The model under review builds one solid part; all positions refer to its coordinate system, in mm. A direction names the side the tool comes from. Round coordinates to 2 decimals unless told otherwise and drop trailing zeros. Order: outer loops, then holes, each group sorted by start corner. A loop starts at its lowest first (then second) coordinate and runs counter-clockwise, first axis right, second up.
```python
from build123d import *

# Parameters (mm, degrees)
SKETCH1_W           = 50
SKETCH1_H           = 77.4
SKETCH1_R           = 2
BOSS_EXTRUDE1_DEPTH = 4
SKETCH2_W           = 50
SKETCH2_H           = 7.168288369
BOSS_EXTRUDE2_DEPTH = 60
SKETCH6_W           = 20
SKETCH6_H           = 26
CUT_EXTRUDE1_DEPTH  = 124.730240351
RIB1_REACH          = 97.821
SKETCH7_WALL_W      = 250.948466038
SKETCH7_WALL_H      = 14
FILLET2_R           = 2
FILLET3_R           = 12
SKETCH8_W           = 13
SKETCH8_H           = 7.168288369
BOSS_EXTRUDE3_DEPTH = 20
FILLET4_R           = 4
BOSS_EXTRUDE4_DEPTH = 6
FILLET5_R           = 2


with BuildPart() as part:
    # Sketch1 → Boss-Extrude1 (new body)
    with BuildSketch(Plane.ZY.offset(8)):
        with Locations((55.110705908, 0)):
            Rectangle(SKETCH1_W, SKETCH1_H)
        with Locations((34.110705908, 33.7)):
            Circle(SKETCH1_R, mode=Mode.SUBTRACT)
        with Locations((41.110705908, 33.7)):
            Circle(SKETCH1_R, mode=Mode.SUBTRACT)
        with Locations((69.110705908, 33.7)):
            Circle(SKETCH1_R, mode=Mode.SUBTRACT)
        with Locations((76.110705908, 33.7)):
            Circle(SKETCH1_R, mode=Mode.SUBTRACT)
        with Locations(Location((34.110705908, -33.7, 0), (0, 0, 180))):
            Circle(SKETCH1_R, mode=Mode.SUBTRACT)
        with Locations(Location((41.110705908, -33.7, 0), (0, 0, 180))):
            Circle(SKETCH1_R, mode=Mode.SUBTRACT)
        with Locations(Location((69.110705908, -33.7, 0), (0, 0, 180))):
            Circle(SKETCH1_R, mode=Mode.SUBTRACT)
        with Locations(Location((76.110705908, -33.7, 0), (0, 0, 180))):
            Circle(SKETCH1_R, mode=Mode.SUBTRACT)
    extrude(amount=BOSS_EXTRUDE1_DEPTH)

    # Sketch2 → Boss-Extrude2 (add)
    with BuildSketch(Plane.ZY.offset(12)):
        with Locations((55.110705908, -25.772954127)):
            Rectangle(SKETCH2_W, SKETCH2_H)
    extrude(amount=BOSS_EXTRUDE2_DEPTH)

    # Sketch6 → Cut-Extrude1 (cut, through all)
    with BuildSketch(Plane(origin=(0, -22.188809942, 0), x_dir=(1, 0, 0), z_dir=(0, 1, 0))):
        with Locations((-22, -43.110705908)):
            Rectangle(SKETCH6_W, SKETCH6_H)
    extrude(amount=-CUT_EXTRUDE1_DEPTH, mode=Mode.SUBTRACT)

    # Sketch7 wall → Rib1 (add, up to next)
    with BuildSketch(Plane(origin=(-26, 2.811190058, 80.110705908), x_dir=(0.488603368932, 0.87250601595, 0), z_dir=(-0.87250601595, 0.488603368932, 0)), mode=Mode.PRIVATE) as rib1_sk1:
        with Locations((0, 7)):
            Rectangle(SKETCH7_WALL_W, SKETCH7_WALL_H)
    rib1_tool1 = extrude(rib1_sk1.sketch, amount=-RIB1_REACH, mode=Mode.PRIVATE) - part.part
    add(rib1_tool1.solids().sort_by_distance((-26, 2.811190058, 80.110705908))[0])

    # Fillet2
    fillet2_edges = [part.edges().sort_by_distance(p)[0] for p in [
        (-12, -29.357098311, 68.110705908),
    ]]
    fillet(fillet2_edges, radius=FILLET2_R)

    # Fillet3
    fillet3_edges = [part.edges().sort_by_distance(p)[0] for p in [
        (-32, -25.772954126, 56.110705908),
    ]]
    fillet(fillet3_edges, radius=FILLET3_R)

    # Sketch8 → Boss-Extrude3 (add)
    with BuildSketch(Plane(origin=(-32, 0, 0), x_dir=(0, 0, -1), z_dir=(1, 0, 0))):
        with Locations((-36.610705908, -25.772954127)):
            Rectangle(SKETCH8_W, SKETCH8_H)
    extrude(amount=BOSS_EXTRUDE3_DEPTH)

    # Fillet4
    fillet4_edges = [part.edges().sort_by_distance(p)[0] for p in [
        (-32, -25.772954126, 43.110705908),
    ]]
    fillet(fillet4_edges, radius=FILLET4_R)

    # Sketch9 → Boss-Extrude4 (add)
    with BuildSketch(Plane(origin=(0, 0, 30.110705908), x_dir=(-1, 0, 0), z_dir=(0, 0, -1))):
        Polygon((42, -22.188809942), (12, 27.811190058), (12, -22.188809942), align=None)
    extrude(amount=-BOSS_EXTRUDE4_DEPTH)

    # Fillet5
    fillet5_edges = [part.edges().sort_by_distance(p)[0] for p in [
        (-12, -29.357098311, 36.610705908),
    ]]
    fillet(fillet5_edges, radius=FILLET5_R)


solid = part.part
```
(1) Draft analysis for pull direction X (two halves, no side actions). For faces 1 (the flat face through (-20, -26, 43.111)), 2 (the flat face through (-26, -11, 30.111)), 3 (the cylindrical face through (-12.57, -29.96, 36.52)), state which applies: pulls with the +X half, pulls with the -X half, needs draft (parallel to the pull), parting line crosses it, or undercut.
Data:
face 1: undercut
face 2: needs draft
face 3: pulls with the -X half
(2) Insertion check: pin 1 (8 mm diameter, centred on x = -29, z = 43.5, fed in from -Y); pin 2 (25 mm diameter, centred on x = -29, z = 67.5, fed in from +Y); pin 3 (5 mm diameter, centred on y = -33.7, z = 34.11, fed in from -X). Each pin has a flat end and moves straight along its axis. Give the tip position at first contact, or say it passes through.
Data:
pin 1: stops at y = -29.36
pin 2: stops at y = 19.78
pin 3: stops at x = -12.01
(3) Consider section C-C (z = 62). Write out the cut boundary in (x, y).
Data:
outline: (-72, -29.36) - (-14, -29.36) arc R2 cw to (-12, -31.36) - (-12, -38.7) - (-8, -38.7) - (-8, 38.7) - (-12, 38.7) - (-12, -22.19) - (-72, -22.19) - close
(4) Consider section B-B (x = -23). Write out the cut boundary in (y, z).
Data:
outline: (-29.36, 30.11) - (9.48, 30.11) - (9.48, 36.11) - (-22.19, 36.11) - (-22.19, 43.11) - (-29.36, 43.11) - close; (-29.36, 55.73) - (-22.19, 55.73) - (-22.19, 66.11) - (8.17, 66.11) - (8.17, 80.11) - (-29.36, 80.11) - close
(5) To check wall thickness, follow probe 1 along Z at (x, y) = (-9.6, -33.7); probe 2 along X at (y, z) = (13.5, 64); probe 3 along Y at (x, z) = (-48.5, 65). State the ranges of each line that lie inside material, in increasing order.
Data:
probe 1: z = 30.11 to 32.11, 36.11 to 39.11, 43.11 to 67.11, 71.11 to 74.11, 78.11 to 80.11
probe 2: x = -12 to -8
probe 3: y = -29.36 to -22.19
(6) Consider section A-A (y = -33.7). Write out the cut boundary in (x, z), and give its area (3 significant figures).
Data:
outline: (-12, 30.11) - (-8, 30.11) - (-8, 32.11) - (-12, 32.11) - close; (-12, 36.11) - (-8, 36.11) - (-8, 39.11) - (-12, 39.11) - close; (-12, 43.11) - (-8, 43.11) - (-8, 67.11) - (-12, 67.11) - close; (-12, 71.11) - (-8, 71.11) - (-8, 74.11) - (-12, 74.11) - close; (-12, 78.11) - (-8, 78.11) - (-8, 80.11) - (-12, 80.11) - close
area: 136 mm2
(7) For faces 4 (the cylindrical face through (-26.8, -25.8, 54)), 5 (the flat face through (-49, -22.189, 55)), 6 (the flat face through (-43, -29.357, 55)), list the 3-axis set-ups (+Z, -Z, +X, -X, +Y, -Y) from which the entire face can be reached by the end or side of a thin tool; tool diameter is ignored.
Data:
face 4: +Y, -Y
face 5: -X, +Y
face 6: +Z, -Z, -X, -Y
(8) Consider section D-D (z = 76.5). Write out the cut boundary in (x, y).
Data:
outline: (-72, -29.36) - (-14, -29.36) arc R2 cw to (-12, -31.36) - (-12, -31.74) - (-8, -31.74) - (-8, 31.74) - (-12, 31.74) - (-12, 27.81) - (-40, -22.19) - (-72, -22.19) - close; (-12, -38.7) - (-8, -38.7) - (-8, -35.66) - (-12, -35.66) - close; (-12, 35.66) - (-8, 35.66) - (-8, 38.7) - (-12, 38.7) - close
